from build123d import *

# Parameters (mm, degrees)
F0_R     = 14.9225
F0_R_2   = 6.1595
F1_DEPTH = 5.461
F2_R     = 1.905
F3_DEPTH = 25.4
F5_ANGLE = 45
F6_R     = 1.905
F7_DEPTH = 5.08


with BuildPart() as f1:
    # F0 (on Top) → F1 (new body)
    with BuildSketch(Plane.XY):
        Circle(F0_R)
        Circle(F0_R_2, mode=Mode.SUBTRACT)
    extrude(amount=F1_DEPTH)

    # F2 (on face) → F3 (cut)
    with BuildSketch(Plane.XY.offset(5.461)):
        with Locations((-11.2395, 0)):
            Circle(F2_R)
        with Locations((0, 11.2395)):
            Circle(F2_R)
        with Locations((11.2395, 0)):
            Circle(F2_R)
        with Locations((0, -11.2395)):
            Circle(F2_R)
    extrude(amount=-F3_DEPTH, mode=Mode.SUBTRACT)


with BuildPart() as f1_1:
    # F5: moved
    add(f1.part.rotate(Axis((0, 0, 9.9508911371), (0, 0, 1)), F5_ANGLE))

    # F6 (on face) → F7 (join)
    with BuildSketch(Plane.XY.offset(5.461)):
        with BuildLine():
            ThreePointArc((-14.3762653704, -4.0005), (-14.9225, 0), (-14.3762653704, 4.0005))
            Line((-14.3762653704, 4.0005), (-22.479, 4.0005))
            ThreePointArc((-22.479, 4.0005), (-26.4795, 0), (-22.479, -4.0005))
            Line((-22.479, -4.0005), (-14.3762653704, -4.0005))
        make_face()
        with Locations((-22.479, 0)):
            Circle(F6_R, mode=Mode.SUBTRACT)
        with BuildLine():
            Line((-4.6835285843, 4.0005), (-14.3762653704, 4.0005))
            ThreePointArc((-14.3762653704, 4.0005), (-14.9225, 0), (-14.3762653704, -4.0005))
            Line((-14.3762653704, -4.0005), (-4.6835285843, -4.0005))
            ThreePointArc((-4.6835285843, -4.0005), (-6.1595, 0), (-4.6835285843, 4.0005))
        make_face()
        with BuildLine():
            ThreePointArc((14.9225, 0), (14.7853107211, 2.0188098301), (14.3762653704, 4.0005))
            Line((14.3762653704, 4.0005), (4.6835285843, 4.0005))
            ThreePointArc((4.6835285843, 4.0005), (5.7787383816, 2.1320466617), (6.1595, 0))
            ThreePointArc((6.1595, 0), (5.7787383816, -2.1320466617), (4.6835285843, -4.0005))
            Line((4.6835285843, -4.0005), (14.3762653704, -4.0005))
            ThreePointArc((14.3762653704, -4.0005), (14.7853107211, -2.0188098301), (14.9225, 0))
        make_face()
        with BuildLine():
            Line((22.479, 4.0005), (14.3762653704, 4.0005))
            ThreePointArc((14.3762653704, 4.0005), (14.7853107211, 2.0188098301), (14.9225, 0))
            ThreePointArc((14.9225, 0), (14.7853107211, -2.0188098301), (14.3762653704, -4.0005))
            Line((14.3762653704, -4.0005), (22.479, -4.0005))
            ThreePointArc((22.479, -4.0005), (26.4795, 0), (22.479, 4.0005))
        make_face()
        with Locations((22.479, 0)):
            Circle(F6_R, mode=Mode.SUBTRACT)
        with BuildLine():
            Line((4.0005, 14.3762653704), (4.0005, 22.479))
            ThreePointArc((4.0005, 22.479), (0, 26.4795), (-4.0005, 22.479))
            Line((-4.0005, 22.479), (-4.0005, 14.3762653704))
            ThreePointArc((-4.0005, 14.3762653704), (0, 14.9225), (4.0005, 14.3762653704))
        make_face()
        with Locations((0, 22.479)):
            Circle(F6_R, mode=Mode.SUBTRACT)
        with BuildLine():
            Line((4.0005, 4.6835285843), (4.0005, 14.3762653704))
            ThreePointArc((4.0005, 14.3762653704), (0, 14.9225), (-4.0005, 14.3762653704))
            Line((-4.0005, 14.3762653704), (-4.0005, 4.6835285843))
            ThreePointArc((-4.0005, 4.6835285843), (0, 6.1595), (4.0005, 4.6835285843))
        make_face()
        with BuildLine():
            ThreePointArc((4.0005, -14.3762653704), (0, -14.9225), (-4.0005, -14.3762653704))
            Line((-4.0005, -14.3762653704), (-4.0005, -22.479))
            ThreePointArc((-4.0005, -22.479), (0, -26.4795), (4.0005, -22.479))
            Line((4.0005, -22.479), (4.0005, -14.3762653704))
        make_face()
        with Locations((0, -22.479)):
            Circle(F6_R, mode=Mode.SUBTRACT)
        with BuildLine():
            Line((-4.0005, -4.6835285843), (-4.0005, -14.3762653704))
            ThreePointArc((-4.0005, -14.3762653704), (0, -14.9225), (4.0005, -14.3762653704))
            Line((4.0005, -14.3762653704), (4.0005, -4.6835285843))
            ThreePointArc((4.0005, -4.6835285843), (0, -6.1595), (-4.0005, -4.6835285843))
        make_face()
    extrude(amount=F7_DEPTH)


solid = f1_1.part
Here's how the part is built. I have some questions about the finished solid (model axes, mm). A direction names the side the tool comes from. Coordinates: 2 decimals unless noted, no trailing zeros. Loops run counter-clockwise (first coordinate to the right, second up) from the corner with the lowest first, then second, coordinate; pieces in that order, holes last. Notation, with made-up numbers: (29.25, -30) -> (66.25, -30) arc R13 cw to (66.25, -6) -> close; hole circle Ø8 at (52, 65.25). An arc over 180 degrees is marked (long way). Use one line per item in the form item = value. Start each with the question number.
(1) If we section it at B-B (x = 0): Please give me the cut outline in (y, z), then the cut area to 3 significant figures.
(2) If we section it at A-A (z = 9.5): Please give me the cut outline in (x, y) (1 decimal), then the cut area to 3 significant figures.
(3) Please list where these lines run through material, in increasing order: line 1 along X through (y, z) = (7, 3); line 2 along X through (y, z) = (0, 3); line 3 along Y through (x, z) = (-20, 10).
(4) If we section it at C-C (y = 7.5): Please give me the cut outline in (x, z), then the cut area to 3 significant figures.
(5) We'd pull the mould along X, two halves only. Please class faces 6 (the face through (-6.13, -8.52, 2.77)), 7 (the face through (-4, -13, 8)), 8 (the face through (-7.8, 10, 5.461)): pulls with the +X half, pulls with the -X half, needs draft (parallel to the pull), parting line crosses it, or undercut.
(6) On a 3-axis mill with a long thin cutter (end or side, diameter ignored), from which of +Z, -Z, +X, -X, +Y, -Y can I reach the whole of each face in a straight line? I mean faces 1 (the face through (-14.91, -0.65, 2.69)), 2 (the face through (14, 4, 8)), 3 (the face through (9, 10, 5.461)), 4 (the face through (-14, -4, 8)), 5 (the face through (6.54, -9.23, 2.77)). Say none if no direction works.
(7) If we section it at D-D (x = -8.5): Please give me the cut outline in (y, z), then the cut area to 3 significant figures.
(8) Will these pins go through, and if not, where does the flat tip stop? pin 1 (5.5 mm diameter, centred on x = -12, z = 7, fed in from +Y); pin 2 (2.5 mm diameter, centred on x = 18, y = -0.5, fed in from -Z); pin 3 (4.5 mm diameter, centred on x = -7.95, y = 7.95, fed in from -Z); pin 4 (2.5 mm diameter, centred on x = 11, z = 8.5, fed in from -Y).
Verdict:
q1.outline = (-26.48, 5.46) -> (-24.38, 5.46) -> (-24.38, 10.54) -> (-26.48, 10.54) -> close; (-20.57, 5.46) -> (-14.92, 5.46) -> (-14.92, 0) -> (-6.16, 0) -> (-6.16, 10.54) -> (-20.57, 10.54) -> close; (6.16, 0) -> (14.92, 0) -> (14.92, 5.46) -> (20.57, 5.46) -> (20.57, 10.54) -> (6.16, 10.54) -> close; (24.38, 5.46) -> (26.48, 5.46) -> (26.48, 10.54) -> (24.38, 10.54) -> close
q1.area = 263 mm²
q2.outline = (-22.5, -4) -> (-4.7, -4) arc R6.2 cw to (-4.7, 4) -> (-22.5, 4) arc R4 ccw to start; (-4, -22.5) arc R4 ccw to (4, -22.5) -> (4, -4.7) arc R6.2 cw to (-4, -4.7) -> close; (-4, 4.7) arc R6.2 cw to (4, 4.7) -> (4, 22.5) arc R4 ccw to (-4, 22.5) -> close; (4.7, -4) -> (22.5, -4) arc R4 ccw to (22.5, 4) -> (4.7, 4) arc R6.2 cw to start; hole circle Ø3.8 at (-22.5, 0); hole circle Ø3.8 at (0, -22.5); hole circle Ø3.8 at (0, 22.5); hole circle Ø3.8 at (22.5, 0)
q2.area = 592 mm²
q3.line_1 = -13.18 to -9.6, -6.29 to 6.29, 9.6 to 13.18
q3.line_2 = -14.92 to -6.16, 6.16 to 14.92
q3.line_3 = -4 to 4
q4.outline = (-12.9, 0) -> (-9.8, 0) -> (-9.8, 5.46) -> (-12.9, 5.46) -> close; (-6.1, 0) -> (6.1, 0) -> (6.1, 5.46) -> (4, 5.46) -> (4, 10.54) -> (-4, 10.54) -> (-4, 5.46) -> (-6.1, 5.46) -> close; (9.8, 0) -> (12.9, 0) -> (12.9, 5.46) -> (9.8, 5.46) -> close
q4.area = 141 mm²
q5.face_6 = undercut
q5.face_7 = pulls with the -X half
q5.face_8 = needs draft
q6.face_1 = -Z
q6.face_2 = +Z, +X, -X, +Y
q6.face_3 = +Z, +X, +Y
q6.face_4 = +Z, +X, -X, -Y
q6.face_5 = +Z, -Z
q7.outline = (-12.27, 0) -> (-9.77, 0) -> (-9.77, 5.46) -> (-12.27, 5.46) -> close; (-6.12, 0) -> (6.12, 0) -> (6.12, 5.46) -> (4, 5.46) -> (4, 10.54) -> (-4, 10.54) -> (-4, 5.46) -> (-6.12, 5.46) -> close; (9.77, 0) -> (12.27, 0) -> (12.27, 5.46) -> (9.77, 5.46) -> close
q7.area = 135 mm²
q8.pin_1 = 11.32
q8.pin_2 = 5.46
q8.pin_3 = 0
q8.pin_4 = -4
